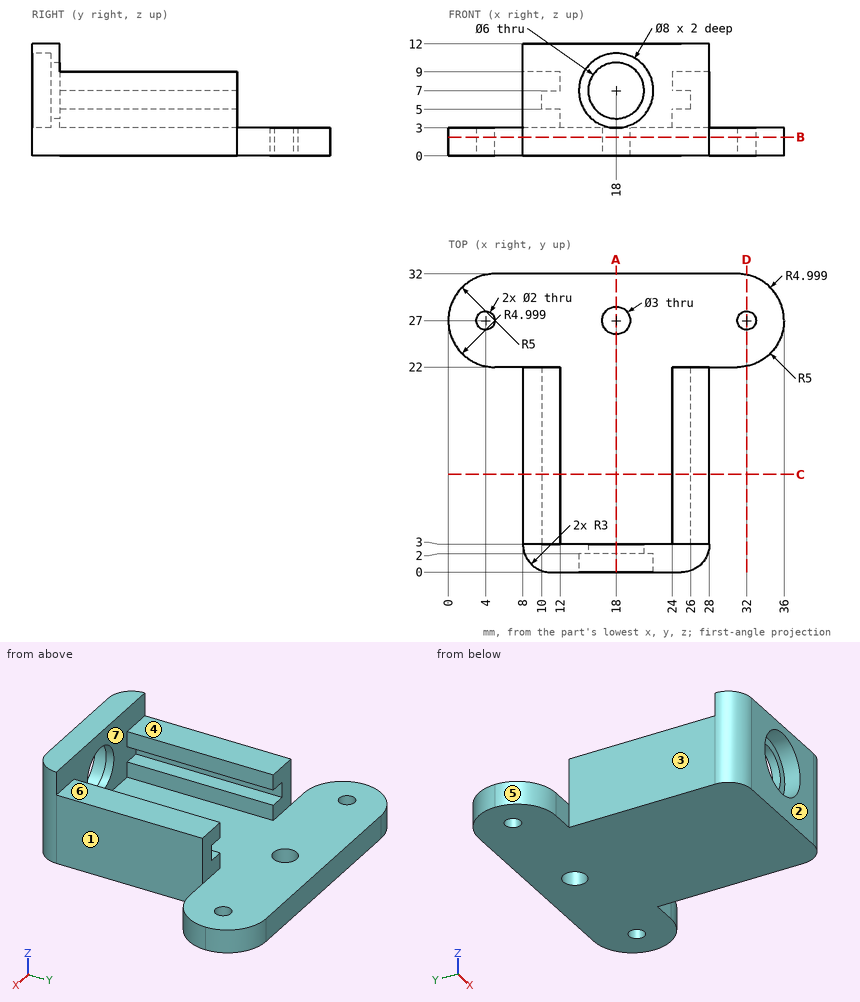
Design review of the part shown in the three views and the two pictorial views. Dimensions are in mm from the part's minimum x, y and z. A direction names the side the tool comes from. Coordinates: 2 decimals unless noted, no trailing zeros. Loops run counter-clockwise (first coordinate to the right, second up) from the corner with the lowest first, then second, coordinate; pieces in that order, holes last. Notation, with made-up numbers: (40, 24) - (91, 24) arc R38 cw to (91, 63) - close; hole circle Ø10 at (71, 63). An arc over 180 degrees is marked (long way). Use a Markdown table: item, result. Add a question column.
Item 1: Insertion check: pin 1 Ø10 at (x, y) = (12.5, 5.5) entering from +Z; pin 2 Ø3.5 at (x, z) = (7, 1) entering from -Y; pin 3 Ø1 at (y, z) = (11, 7.5) entering from -X; pin 4 Ø3 at (x, y) = (27, 16.5) entering from +Z. Each pin has a flat end and moves straight along its axis. Give the tip position at first contact, or say it passes through.
Item 2: We need section B-B (z = 2). Give the number of separate pieces and of enclosed holes in the cut face, and give its area (3 significant figures).
Item 3: We need section C-C (y = 10.5). Give the boundary of the cut face in (x, z).
Item 4: For line 1 (X direction, y = 27, z = 1.35); line 2 (Y direction, x = 18, z = 1.3); line 3 (Z direction, x = 18, y = 1.35), list the stretches that pass through material, from the lowest coordinate up.
Item 5: We need section D-D (x = 32). Give the boundary of the cut face in (y, z).
Item 6: Tool access review of the marked faces 1, 2, 3 and 4: name each direction out of +Z, -Z, +X, -X, +Y, -Y from which nothing blocks a thin tool from reaching the whole face with its end or side.
Item 7: We need section A-A (x = 18). Give the boundary of the cut face in (y, z), and give its area (3 significant figures).
Item 8: Mouldability with a two-part tool opening along X and no side actions: class the marked faces 5, 6 and 7 as pulls with the +X half, pulls with the -X half, needs draft (parallel to the pull), parting line crosses it, or undercut.
Results list:
| question | item | result |
|---|---|---|
| 1 | pin 1 | stops at z = 12 |
| 1 | pin 2 | stops at y = 1.02 |
| 1 | pin 3 | stops at x = 8 |
| 1 | pin 4 | stops at z = 9 |
| 2 | separate pieces | 1 |
| 2 | enclosed holes | 3 |
| 2 | area | 761 mm^2 |
| 3 | outline | (8, 0) - (28, 0) - (28, 9) - (24, 9) - (24, 7) - (26, 7) - (26, 5) - (24, 5) - (24, 3) - (12, 3) - (12, 5) - (10, 5) - (10, 7) - (12, 7) - (12, 9) - (8, 9) - close |
| 4 | line 1 | x = 0 to 3, 5 to 16.5, 19.5 to 31, 33 to 36 |
| 4 | line 2 | y = 0 to 25.5, 28.5 to 32 |
| 4 | line 3 | z = 0 to 3, 11 to 12 |
| 5 | outline | (22.1, 0) - (26, 0) - (26, 3) - (22.1, 3) - close; (28, 0) - (31.9, 0) - (31.9, 3) - (28, 3) - close |
| 6 | face 1 | +Z, -Z, +X, -Y |
| 6 | face 2 | +Z, -Z, +X, -X, -Y |
| 6 | face 3 | +Z, -Z, -X, -Y |
| 6 | face 4 | +Z, +X, -X, +Y |
| 7 | outline | (0, 0) - (25.5, 0) - (25.5, 3) - (3, 3) - (3, 4) - (2, 4) - (2, 3) - (0, 3) - close; (0, 11) - (2, 11) - (2, 10) - (3, 10) - (3, 12) - (0, 12) - close; (28.5, 0) - (32, 0) - (32, 3) - (28.5, 3) - close |
| 7 | area | 92.0 mm^2 |
| 8 | face 5 | pulls with the -X half |
| 8 | face 6 | needs draft |
| 8 | face 7 | undercut |
